from build123d import *

# Parameters (mm, degrees)
EXTRUDE_1_DEPTH     = 3.6
SKETCH_2_R          = 3.25
SKETCH_2_R_2        = 2
EXTRUDE_2_DEPTH     = 1.05
SKETCH_3_R          = 2
CUT_EXTRUDE_1_DEPTH = 7.306734496
FILLET_1_R          = 0.2
FILLET_2_R          = 0.2


with BuildPart() as part:
    # 草图1 → 凸台-拉伸1 (new body)
    with BuildSketch(Plane.XY):
        Polygon((-3.39, -1.957217413), (0, -3.914434825), (3.39, -1.957217413), (3.39, 1.957217413), (0, 3.914434825), (-3.39, 1.957217413), align=None)
    extrude(amount=EXTRUDE_1_DEPTH)

    # 草图2 → 凸台-拉伸2 (add)
    with BuildSketch(Plane.XY.offset(3.6)):
        Circle(SKETCH_2_R)
        Circle(SKETCH_2_R_2, mode=Mode.SUBTRACT)
    extrude(amount=EXTRUDE_2_DEPTH)

    # 草图3 → 切除-拉伸1 (cut, through all)
    with BuildSketch(Plane.XY.offset(3.6)):
        Circle(SKETCH_3_R)
    extrude(amount=-CUT_EXTRUDE_1_DEPTH, mode=Mode.SUBTRACT)

    # 圆角1
    fillet_1_edges = [part.edges().sort_by_distance(p)[0] for p in [
        (-2, 0, 4.65),
    ]]
    fillet(fillet_1_edges, radius=FILLET_1_R)

    # 圆角2
    fillet_2_edges = [part.edges().sort_by_distance(p)[0] for p in [
        (-3.25, 0, 4.65),
    ]]
    fillet(fillet_2_edges, radius=FILLET_2_R)


solid = part.part
Can you work these out from the model? Positions are in its coordinate system, mm. A direction names the side the tool comes from. Give positions to 0.01 mm unless a question says otherwise; leave off trailing zeros. Write each loop counter-clockwise with the first axis right and the second up, starting at its lowest first coordinate (ties: lowest second). Pieces come first, ordered by that corner, then holes. Notation, with made-up numbers: M 11.25,27.5 L 36.25,27.5 A23 cw 36.25,59.5 Z; hole C 18,17.5 d6. An arc over 180 degrees is marked long. Answer in a Markdown table with one row per item. Add a question column.
Item 1: Please list where these lines run through material, in increasing order: L1, parallel to Y at x = 0, z = 3.95; L2, parallel to Y at x = 1.5, z = 4.3; L3, parallel to X at y = 0.5, z = 2.3.
Item 2: Imagine slicing it at B-B, the plane z = 2. Write out the boundary of the cut face in (x, y).
Item 3: On a 3-axis mill with a long thin cutter (end or side, diameter ignored), from which of +Z, -Z, +X, -X, +Y, -Y can I reach the whole of each face in a straight line? I mean faces 1 (the cylindrical face through (-2.579, -1.978, 4.019)), 2 (the flat face through (3.39, 0, 2)). Say none if no direction works.
Item 4: Imagine slicing it at C-C, the plane z = 3.9. Write out the boundary of the cut face in (x, y), plus the area to 3 significant figures.
Item 5: Imagine slicing it at A-A, the plane y = 0. Write out the boundary of the cut face in (x, z).
Item 6: For pin 1 Ø1 at (y, z) = (2, 3.5) entering from +X; pin 2 Ø1 at (x, z) = (1, 0.5) entering from +Y; pin 3 Ø2 at (x, z) = (-2, 0.5) entering from +Y, each with a flat end and sliding along its axis, tell me the tip position at first contact or that it passes through.
Evaluation:
| question | item | result |
|---|---|---|
| 1 | L1 | y = -3.25 to -2, 2 to 3.25 |
| 1 | L2 | y = -2.88 to -1.32, 1.32 to 2.88 |
| 1 | L3 | x = -3.39 to -1.94, 1.94 to 3.39 |
| 2 | outline | M -3.39,-1.96 L 0,-3.91 L 3.39,-1.96 L 3.39,1.96 L 0,3.91 L -3.39,1.96 Z; hole C 0,0 d4 |
| 3 | face 1 | +Z |
| 3 | face 2 | +Z, -Z, +X, +Y, -Y |
| 4 | outline | C 0,0 d6.5; hole C 0,0 d4 |
| 4 | area | 20.6 mm² |
| 5 | outline | M -3.39,0 L -2,0 L -2,4.45 A0.2 ccw -2.2,4.65 L -3.05,4.65 A0.2 ccw -3.25,4.45 L -3.25,3.6 L -3.39,3.6 Z; M 2,0 L 3.39,0 L 3.39,3.6 L 3.25,3.6 L 3.25,4.45 A0.2 ccw 3.05,4.65 L 2.2,4.65 A0.2 ccw 2,4.45 Z |
| 6 | pin 1 | stops at x = 3.39 |
| 6 | pin 2 | stops at y = 3.63 |
| 6 | pin 3 | stops at y = 3.34 |
